```python
from build123d import *

# Parameters (mm, degrees)
SKETCH_1_R          = 1.6
SKETCH_1_W          = 7.387531562
SKETCH_1_H          = 3.94976935
SKETCH_1_W_2        = 20.26085389
SKETCH_1_H_2        = 4.973783626
EXTRUDE_1_DEPTH     = 3
SKETCH_2_W          = 27
SKETCH_2_H          = 1.5
EXTRUDE_2_DEPTH     = 14
SKETCH_4_W          = 27
SKETCH_4_H          = 4
EXTRUDE_3_DEPTH     = 30
SKETCH_5_R          = 1.6
CUT_EXTRUDE_1_DEPTH = 30


with BuildPart() as part:
    # 草图1 → 凸台-拉伸1 (new body)
    with BuildSketch(Plane(origin=(0, 0, 0), x_dir=(1, 0, 0), z_dir=(0, 1, 0))):
        with BuildLine():
            Line((-49.5, -40.220425864), (49.5, -40.220425864))
            ThreePointArc((49.5, -40.220425864), (50.914213562, -39.634639426), (51.5, -38.220425864))
            Line((51.5, -38.220425864), (51.5, 38.220425864))
            ThreePointArc((51.5, 38.220425864), (50.914213562, 39.634639426), (49.5, 40.220425864))
            Line((49.5, 40.220425864), (20.187430173, 40.220425864))
            Line((20.187430173, 40.220425864), (20.187430173, 26.249140852))
            Line((20.187430173, 26.249140852), (-20.187430173, 26.249140852))
            Line((-20.187430173, 26.249140852), (-20.187430173, 40.220425864))
            Line((-20.187430173, 40.220425864), (-49.5, 40.220425864))
            ThreePointArc((-49.5, 40.220425864), (-50.914213562, 39.634639426), (-51.5, 38.220425864))
            Line((-51.5, 38.220425864), (-51.5, -38.220425864))
            ThreePointArc((-51.5, -38.220425864), (-50.914213562, -39.634639426), (-49.5, -40.220425864))
        make_face()
        with Locations(Location((-43.3, -32.020425864, 0), (0, 0, 270))):
            Circle(SKETCH_1_R, mode=Mode.SUBTRACT)
        with Locations((-37.047373629, -33.829043047)):
            Rectangle(SKETCH_1_W, SKETCH_1_H, mode=Mode.SUBTRACT)
        with Locations((0.109715815, -31.854158372)):
            Rectangle(SKETCH_1_W_2, SKETCH_1_H_2, mode=Mode.SUBTRACT)
        with Locations((37.047373629, -33.829043047)):
            Rectangle(SKETCH_1_W, SKETCH_1_H, mode=Mode.SUBTRACT)
        with Locations(Location((43.3, -32.020425864, 0), (0, 0, 270))):
            Circle(SKETCH_1_R, mode=Mode.SUBTRACT)
        with Locations(Location((43.3, 32.020425864, 0), (0, 0, 270))):
            Circle(SKETCH_1_R, mode=Mode.SUBTRACT)
        with Locations(Location((-43.3, 32.020425864, 0), (0, 0, 270))):
            Circle(SKETCH_1_R, mode=Mode.SUBTRACT)
    extrude(amount=EXTRUDE_1_DEPTH)

    # 草图2 → 凸台-拉伸2 (add)
    with BuildSketch(Plane.XY.offset(40.220425864)):
        with Locations((-19.346509013, 0.75)):
            Rectangle(SKETCH_2_W, SKETCH_2_H)
    extrude(amount=EXTRUDE_2_DEPTH)

    # 草图4 → 凸台-拉伸3 (add)
    with BuildSketch(Plane(origin=(0, 1.5, 0), x_dir=(1, 0, 0), z_dir=(0, 1, 0))):
        with Locations((-19.346509013, -52.220425864)):
            Rectangle(SKETCH_4_W, SKETCH_4_H)
    extrude(amount=EXTRUDE_3_DEPTH)

    # 草图5 → 切除-拉伸1 (cut)
    with BuildSketch(Plane.XY.offset(54.220425864)):
        with Locations((-29.596509013, 28.381274353)):
            Circle(SKETCH_5_R)
        with Locations((-9.096509013, 28.381274353)):
            Circle(SKETCH_5_R)
    extrude(amount=-CUT_EXTRUDE_1_DEPTH, mode=Mode.SUBTRACT)


solid = part.part
```
Read the model definition and answer for the solid it produces. Units are mm, in the model's axes. A direction names the side the tool comes from. Give positions to 0.01 mm unless a question says otherwise; leave off trailing zeros. Order: outer loops, then holes, each group sorted by start corner. A loop starts at its lowest first (then second) coordinate and runs counter-clockwise, first axis right, second up. Notation, with made-up numbers: (53, 3.5) -> (108, 3.5) arc R23 cw to (108, 33.5) -> close; hole circle Ø9 at (-8.75, -35). An arc over 180 degrees is marked (long way). One line per item, written item: value. Start each with the question number.
(1) The part is cut by section D-D (z = -25). Determine the outline of the cut face in (x, y).
(2) Straight lines are drawn through the part: L1, parallel to Z at x = -43, y = 1; L2, parallel to Y at x = 44, z = 26; L3, parallel to Z at x = -21, y = 26. For each, find the intervals that lie inside material, in ascending order.
(3) A tool of negligible diameter and unlimited length cuts with its end or side. For faces 1 (the flat face through (-5.847, 15, 51)), 2 (the flat face through (33.354, 1, 34)), 3 (the flat face through (-20.187, 1, -33)), 4 (the flat face through (-1, 3, -1)), from which of +Z, -Z, +X, -X, +Y, -Y can it reach the whole face along a straight path? Write none if from no direction.
(4) The part is cut by section B-B (x = -19). Determine the outline of the cut face in (y, z), and give its area (3 significant figures).
(5) Flat-ended cylindrical pins translate along their axes: P1, Ø4, axis at y = 11.5, z = 48, coming from the -X side; P2, Ø3.5, axis at x = -29.6, y = 28.38, coming from the -Z side; P3, Ø0.9, axis at x = -4.5, y = 1, coming from the +Z side; P4, Ø15.5, axis at y = 20, z = 45, coming from the +X side. Find the tip coordinate at first contact, or state that the pin passes through.
(6) The part is cut by section A-A (x = 43.3). Determine the outline of the cut face in (y, z), and give its area (3 significant figures).
(7) For a pull along Z with two mould halves and no side action, classify faces 5 (the cylindrical face through (-28.86, 26.96, 52.25)), 6 (the flat face through (-35, 1, -40.22)), 7 (the flat face through (-40.741, 1, 34)) as released by +Z, released by -Z, zero draft, split by the parting line, or undercut.
(8) The part is cut by section C-C (y = 13). Determine the outline of the cut face in (x, z), and give its area (3 significant figures).
Taken from the geometry:
1. outline: (-51.5, 0) -> (51.5, 0) -> (51.5, 3) -> (-51.5, 3) -> close
2. L1: -40.22 to -33.59, -30.45 to 30.45, 33.59 to 40.22
2. L2: 0 to 3
2. L3: 50.22 to 54.22
3. face 1: +Z, +X, +Y, -Y
3. face 2: +Y, -Y
3. face 3: -Z, +Y, -Y
3. face 4: -Z, +X, -X, +Y
4. outline: (0, -26.25) -> (3, -26.25) -> (3, 40.22) -> (1.5, 40.22) -> (1.5, 50.22) -> (31.5, 50.22) -> (31.5, 54.22) -> (0, 54.22) -> close
4. area: 340 mm^2
5. P1: through
5. P2: z = 50.22
5. P3: z = 40.22
5. P4: x = -5.85
6. outline: (0, -40.22) -> (3, -40.22) -> (3, -33.62) -> (0, -33.62) -> close; (0, -30.42) -> (3, -30.42) -> (3, 30.42) -> (0, 30.42) -> close; (0, 33.62) -> (3, 33.62) -> (3, 40.22) -> (0, 40.22) -> close
6. area: 222 mm^2
7. face 5: zero draft
7. face 6: released by -Z
7. face 7: undercut
8. outline: (-32.85, 50.22) -> (-5.85, 50.22) -> (-5.85, 54.22) -> (-32.85, 54.22) -> close
8. area: 108 mm^2
